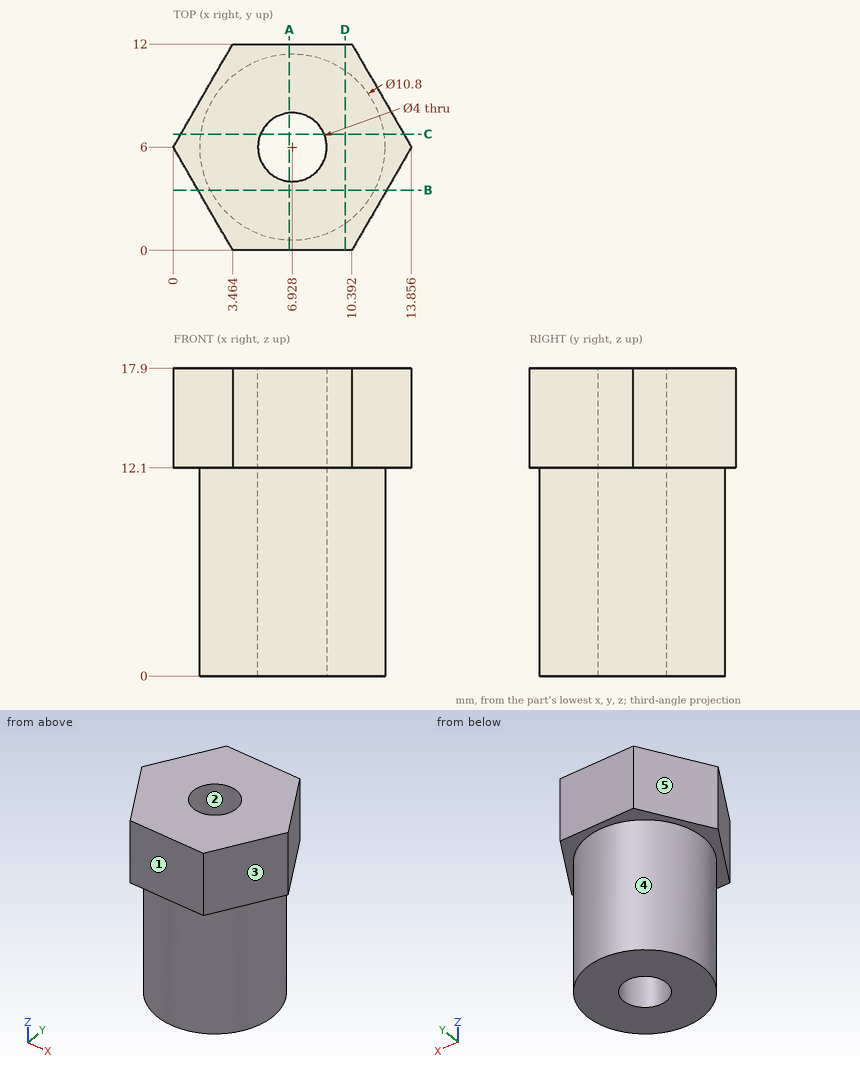
Print and shaded views of the part. All mm, measured from the part's lowest x, y and z. A direction names the side the tool comes from. Give positions to 0.01 mm unless a question says otherwise; leave off trailing zeros. Loops run counter-clockwise (first coordinate to the right, second up) from the corner with the lowest first, then second, coordinate; pieces in that order, holes last.
1) Saw through at C-C (y = 6.75). Write the cut outline in (x, z), plus the area to 3 significant figures.
2) Saw through at A-A (x = 6.75). Write the cut outline in (y, z), plus the area to 3 significant figures.
3) Wall check: line 1 (X direction, y = 7, z = 7.75) (1 decimal); line 2 (X direction, y = 6.75, z = 2.25) (1 decimal); line 3 (Y direction, x = 7, z = 1.5). Give the ranges that are in metal, low to high.
4) Pull direction X, two halves, no side cores. Call the marked faces 1, 2 and 3: +X half, -X half, draft (parallel to the pull), parting line (faces both ways), or undercut.
5) Saw through at B-B (y = 3.5). Write the cut outline in (x, z) (1 decimal).
6) Flat gauge pins, fed straight in: pin 1 Ø3 at (y, z) = (6, 3) entering from +X; pin 2 Ø4 at (x, z) = (8.5, 7.5) entering from +Y. Where does each tip first touch, or does it go through?
7) Saw through at D-D (x = 10). Write the cut outline in (y, z), plus the area to 3 significant figures.
8) Tool access for the marked faces 4 and 5: list every direction of +Z, -Z, +X, -X, +Y, -Y with a clear straight run to the whole face (end or side of a thin tool).
Answer block:
1. outline: (0.43, 12.1) - (1.58, 12.1) - (1.58, 0) - (5.07, 0) - (5.07, 17.9) - (0.43, 17.9) - close; (8.78, 0) - (12.28, 0) - (12.28, 12.1) - (13.42, 12.1) - (13.42, 17.9) - (8.78, 17.9) - close
1. area: 138 mm2
2. outline: (0, 12.1) - (0.6, 12.1) - (0.6, 0) - (4.01, 0) - (4.01, 17.9) - (0, 17.9) - close; (7.99, 0) - (11.4, 0) - (11.4, 12.1) - (12, 12.1) - (12, 17.9) - (7.99, 17.9) - close
2. area: 129 mm2
3. line 1: x = 1.6 to 5.2, 8.7 to 12.2
3. line 2: x = 1.6 to 5.1, 8.8 to 12.3
3. line 3: y = 0.6 to 4, 8 to 11.4
4. face 1: draft
4. face 2: undercut
4. face 3: +X half
5. outline: (1.4, 12.1) - (2.1, 12.1) - (2.1, 0) - (11.7, 0) - (11.7, 12.1) - (12.4, 12.1) - (12.4, 17.9) - (1.4, 17.9) - close
6. pin 1: stops at x = 12.33
6. pin 2: stops at y = 11.4
7. outline: (0, 12.1) - (1.56, 12.1) - (1.56, 0) - (10.44, 0) - (10.44, 12.1) - (12, 12.1) - (12, 17.9) - (0, 17.9) - close
7. area: 177 mm2
8. face 4: -Z
8. face 5: +Z, -Z, -X, +Y
